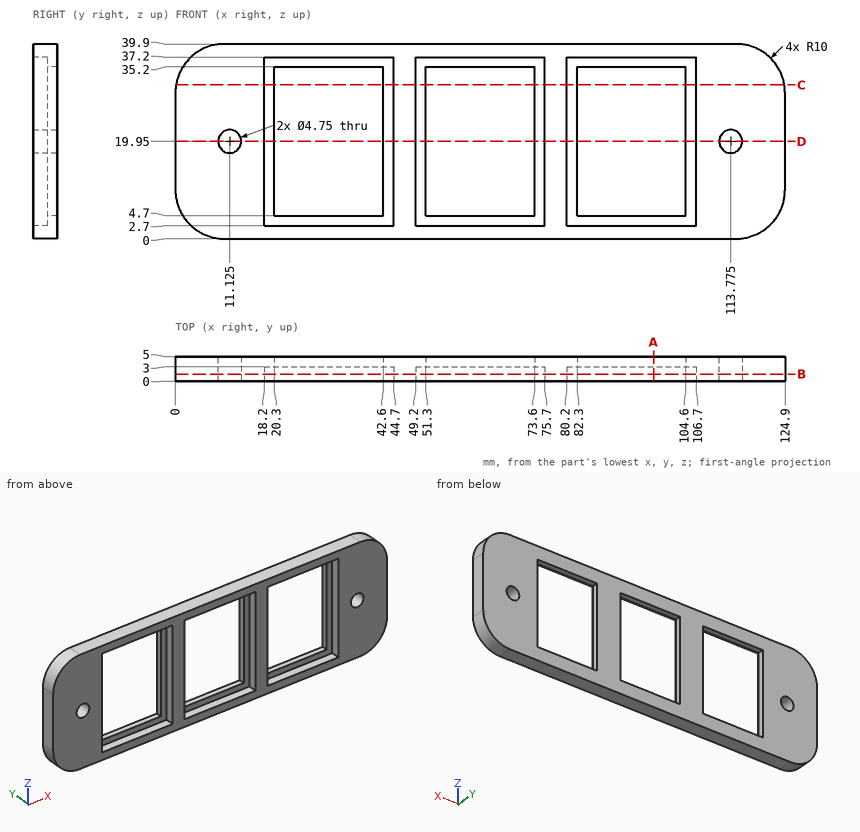
Study the drawing (mm; zero at the part's minimum x, y, z) and answer. Coordinates: 2 decimals unless noted, no trailing zeros. Loops run counter-clockwise (first coordinate to the right, second up) from the corner with the lowest first, then second, coordinate; pieces in that order, holes last. Notation, with made-up numbers: (36.25, 43) -> (60.25, 43) arc R22 ccw to (60.25, 78) -> close; hole circle Ø9 at (-29.5, 14.5). An arc over 180 degrees is marked (long way). Answer in a Markdown table with one row per item. Add a question column.
1. The part is cut by section A-A, the plane x = 98. Write down the section's boundary in (y, z).
2. The part is cut by section D-D, the plane z = 19.95. Count the separate pieces of the cut face and the enclosed holes in it, then the cut area to 3 significant figures.
3. The part is cut by section C-C, the plane z = 31.5. Write down the section's boundary in (x, y), then the cut area to 3 significant figures.
4. The part is cut by section B-B, the plane y = 1.45. Write down the section's boundary in (x, z) (3 decimals).
5. Consider line 1 (X direction, y = 1.6, z = 12.5); line 2 (X direction, y = 4.25, z = 30); line 3 (Z direction, x = 27.5, y = 2.65). Determine where each line is inside the solid, lowest interval first. Write a range as [from, to].
Answer below:
| question | item | result |
|---|---|---|
| 1 | outline | (0, 0) -> (5, 0) -> (5, 4.7) -> (3, 4.7) -> (3, 2.7) -> (0, 2.7) -> close; (0, 37.2) -> (3, 37.2) -> (3, 35.2) -> (5, 35.2) -> (5, 39.9) -> (0, 39.9) -> close |
| 2 | separate pieces | 6 |
| 2 | enclosed holes | 0 |
| 2 | area | 205 mm2 |
| 3 | outline | (0.13, 0) -> (18.2, 0) -> (18.2, 3) -> (20.3, 3) -> (20.3, 5) -> (0.13, 5) -> close; (42.6, 3) -> (44.7, 3) -> (44.7, 0) -> (49.2, 0) -> (49.2, 3) -> (51.3, 3) -> (51.3, 5) -> (42.6, 5) -> close; (73.6, 3) -> (75.7, 3) -> (75.7, 0) -> (80.2, 0) -> (80.2, 3) -> (82.3, 3) -> (82.3, 5) -> (73.6, 5) -> close; (104.6, 3) -> (106.7, 3) -> (106.7, 0) -> (124.77, 0) -> (124.77, 5) -> (104.6, 5) -> close |
| 3 | area | 251 mm2 |
| 4 | outline | (0, 10) arc R10 ccw to (10, 0) -> (114.9, 0) arc R10 ccw to (124.9, 10) -> (124.9, 29.9) arc R10 ccw to (114.9, 39.9) -> (10, 39.9) arc R10 ccw to (0, 29.9) -> close; hole circle Ø4.75 at (11.125, 19.95); hole (18.2, 2.7) -> (44.7, 2.7) -> (44.7, 37.2) -> (18.2, 37.2) -> close; hole (49.2, 2.7) -> (75.7, 2.7) -> (75.7, 37.2) -> (49.2, 37.2) -> close; hole (80.2, 2.7) -> (106.7, 2.7) -> (106.7, 37.2) -> (80.2, 37.2) -> close; hole circle Ø4.75 at (113.775, 19.95) |
| 5 | line 1 | [0, 18.2], [44.7, 49.2], [75.7, 80.2], [106.7, 124.9] |
| 5 | line 2 | [0, 20.3], [42.6, 51.3], [73.6, 82.3], [104.6, 124.9] |
| 5 | line 3 | [0, 2.7], [37.2, 39.9] |
